Read the model definition and answer for the solid it produces. Units are mm, in the model's axes. A direction names the side the tool comes from. Give positions to 0.01 mm unless a question says otherwise; leave off trailing zeros. Order: outer loops, then holes, each group sorted by start corner. A loop starts at its lowest first (then second) coordinate and runs counter-clockwise, first axis right, second up. Notation, with made-up numbers: (7.5, 61.25) - (35.5, 61.25) arc R18 cw to (35.5, 90.25) - close; hole circle Ø5 at (-23, 66). An arc over 180 degrees is marked (long way). Write item = value, one per line.
```python
from build123d import *

# Parameters (mm, degrees)
SKETCH1_R           = 18.5
BOSS_EXTRUDE1_DEPTH = 24
SKETCH2_R           = 18
BOSS_EXTRUDE2_DEPTH = 60
SKETCH3_R           = 6
BOSS_EXTRUDE3_DEPTH = 6
SKETCH4_R           = 3
BOSS_EXTRUDE4_DEPTH = 15
SKETCH5_R           = 2
CUT_EXTRUDE1_DEPTH  = 2


with BuildPart() as part:
    # Sketch1 → Boss-Extrude1 (new body)
    with BuildSketch(Plane(origin=(0, 0, 0), x_dir=(0, 0, -1), z_dir=(1, 0, 0))):
        Circle(SKETCH1_R)
    extrude(amount=-BOSS_EXTRUDE1_DEPTH)

    # Sketch2 → Boss-Extrude2 (add)
    with BuildSketch(Plane.ZY.offset(24)):
        Circle(SKETCH2_R)
    extrude(amount=BOSS_EXTRUDE2_DEPTH)

    # Sketch3 → Boss-Extrude3 (add)
    with BuildSketch(Plane(origin=(0, 0, 0), x_dir=(0, 0, -1), z_dir=(1, 0, 0))):
        with Locations((0, -7)):
            Circle(SKETCH3_R)
    extrude(amount=BOSS_EXTRUDE3_DEPTH)

    # Sketch4 → Boss-Extrude4 (add)
    with BuildSketch(Plane(origin=(6, 0, 0), x_dir=(0, 0, -1), z_dir=(1, 0, 0))):
        with Locations((0, -7)):
            Circle(SKETCH4_R)
    extrude(amount=BOSS_EXTRUDE4_DEPTH)

    # Sketch5 → Cut-Extrude1 (cut)
    with BuildSketch(Plane(origin=(0, 0, 0), x_dir=(0, 0, -1), z_dir=(1, 0, 0))):
        with Locations((-15.5, 0)):
            Circle(SKETCH5_R)
        with Locations((-7.75, 13.423393759)):
            Circle(SKETCH5_R)
        with Locations((7.75, 13.423393759)):
            Circle(SKETCH5_R)
        with Locations((15.5, 0)):
            Circle(SKETCH5_R)
        with Locations((7.75, -13.423393759)):
            Circle(SKETCH5_R)
        with Locations((-7.75, -13.423393759)):
            Circle(SKETCH5_R)
    extrude(amount=-CUT_EXTRUDE1_DEPTH, mode=Mode.SUBTRACT)


solid = part.part
```
1. Section B-B (y = 0) is taken. Determine the outline of the cut face in (x, z), and give its area (3 significant figures).
Recorded:
outline = (-84, -18) - (-24, -18) - (-24, -18.5) - (0, -18.5) - (0, -17.5) - (-2, -17.5) - (-2, -13.5) - (0, -13.5) - (0, 13.5) - (-2, 13.5) - (-2, 17.5) - (0, 17.5) - (0, 18.5) - (-24, 18.5) - (-24, 18) - (-84, 18) - close
area = 3,030 mm^2
2. For faces 4 (the face through (-11.83, -18.06, 4.01)), 5 (the face through (-1, -1.2, -13.9)), 6 (the face through (-24, -17.73, -4.02)), determine the directions among +Z, -Z, +X, -X, +Y, -Y from which every point of the face is accessible in a straight line to the end or side of a thin tool.
Recorded:
face_4 = +X, -X
face_5 = +X
face_6 = -X
3. Flat-ended cylindrical pins translate along their axes: pin 1 (3 mm diameter, centred on y = -0.5, z = 16, fed in from +X); pin 2 (10 mm diameter, centred on x = -63.5, y = 5, fed in from -Z); pin 3 (8 mm diameter, centred on x = -4, y = 11, fed in from +Z); pin 4 (18.5 mm diameter, centred on y = -1, z = -6, fed in from +X). Find the tip coordinate at first contact, or state that the pin passes through.
Recorded:
pin_1 = 0
pin_2 = -18
pin_3 = 17.12
pin_4 = 21
4. Section A-A (z = 0) is taken. Determine the outline of the cut face in (x, y), and give its area (3 significant figures).
Recorded:
outline = (-84, -18) - (-24, -18) - (-24, -18.5) - (0, -18.5) - (0, -13) - (6, -13) - (6, -10) - (21, -10) - (21, -4) - (6, -4) - (6, -1) - (0, -1) - (0, 18.5) - (-24, 18.5) - (-24, 18) - (-84, 18) - close
area = 3,210 mm^2
5. Section C-C (x = -52.5) is taken. Determine the outline of the cut face in (y, z), and give its area (3 significant figures).
Recorded:
outline = circle Ø36 at (0, 0)
area = 1,020 mm^2
6. Determine the mould class of faces 1 (the face through (-2, 13, -8)), 2 (the face through (0, 0, 0)), 3 (the face through (3, -7, 6)) for opening direction Y: +Y half, -Y half, draft (parallel to the pull), parting line (faces both ways), or undercut.
Recorded:
face_1 = undercut
face_2 = draft
face_3 = parting line
7. Straight lines are drawn through the part: L1, parallel to Y at x = -0.95, z = -7.75; L2, parallel to X at y = -16, z = -4.5; L3, parallel to Y at x = -22.5, z = 0. For each, find the intervals that lie inside material, in ascending order. Write a range as [from, to].
Recorded:
L1 = [-16.8, -15.42], [-11.42, 11.42], [15.42, 16.8]
L2 = [-84, 0]
L3 = [-18.5, 18.5]
8. Section D-D (z = -15.5) is taken. Determine the outline of the cut face in (x, y).
Recorded:
outline = (-84, -9.15) - (-24, -9.15) - (-24, -10.1) - (0, -10.1) - (0, -2) - (-2, -2) - (-2, 2) - (0, 2) - (0, 10.1) - (-24, 10.1) - (-24, 9.15) - (-84, 9.15) - close
